The model under review builds one solid part; all positions refer to its coordinate system, in mm. Give positions to 0.01 mm unless a question says otherwise; leave off trailing zeros. Loops run counter-clockwise (first coordinate to the right, second up) from the corner with the lowest first, then second, coordinate; pieces in that order, holes last. Notation, with made-up numbers: M 66,74 L 100,74 A20 ccw 100,105 Z; hole C 30,13.5 d8. An arc over 180 degrees is marked long. One line per item, written item: value. Start each with the question number.
Q1. For pin 1 (1.5 mm diameter, centred on y = 34.5, z = 1.5, fed in from +X), flat-tipped, find the tip position at first contact; note if it passes through.
Q2. We need section A-A on x = 0. Write out the cut boundary in (y, z), plus the area to 3 significant figures.
Q3. We need section D-D on x = -13. Write out the cut boundary in (y, z).
Q4. To check wall thickness, follow line 1 along Y through (x, z) = (0, 2.95); line 2 along X through (y, z) = (-14, 0.55); line 3 along X through (y, z) = (-11.5, 1.2). State the ranges of each line that lie inside material, in increasing order. Write a range as from..to.
Q5. We need section B-B on x = 39. Write out the cut boundary in (y, z), plus the area to 3 significant figures.
Q6. We need section C-C on y = -24.5. Write out the cut boundary in (x, z), plus the area to 3 significant figures.
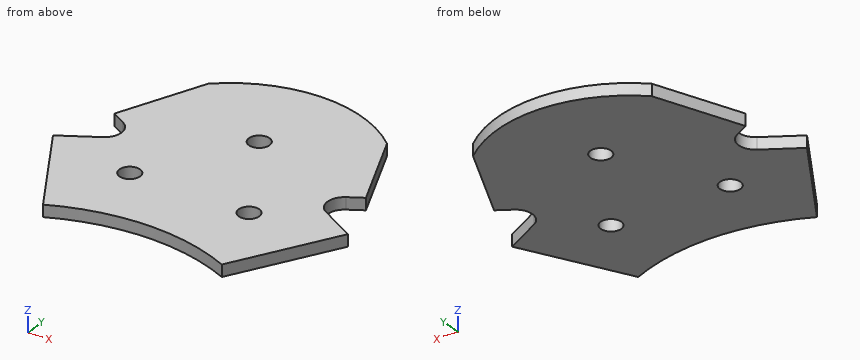
```python
from build123d import *

# Parameters (mm, degrees)
SKETCH1_R           = 3.5
BOSS_EXTRUDE1_DEPTH = 4


with BuildPart() as part:
    # Sketch1 → Boss-Extrude1 (new body)
    with BuildSketch(Plane.XY):
        with BuildLine():
            Line((-30, -39.805989232), (-49.472997898, -6.077767497))
            Line((-49.472997898, -6.077767497), (-37.435244785, 0.872232503))
            ThreePointArc((-37.435244785, 0.872232503), (-34.548493439, 5.872232503), (-37.435244785, 10.872232503))
            Line((-37.435244785, 10.872232503), (-42.198384506, 13.622232503))
            Line((-42.198384506, 13.622232503), (-30, 42.12134504))
            ThreePointArc((-30, 42.12134504), (0, 53.594010768), (30, 42.12134504))
            Line((30, 42.12134504), (42.198384506, 13.622232503))
            Line((42.198384506, 13.622232503), (37.435244785, 10.872232503))
            ThreePointArc((37.435244785, 10.872232503), (34.548493439, 5.872232503), (37.435244785, 0.872232503))
            Line((37.435244785, 0.872232503), (49.472997898, -6.077767497))
            Line((49.472997898, -6.077767497), (30, -39.805989232))
            ThreePointArc((30, -39.805989232), (0, -33.105989232), (-30, -39.805989232))
        make_face()
        with Locations((0, 23.094010768)):
            Circle(SKETCH1_R, mode=Mode.SUBTRACT)
        with Locations((-20, -11.547005384)):
            Circle(SKETCH1_R, mode=Mode.SUBTRACT)
        with Locations((20, -11.547005384)):
            Circle(SKETCH1_R, mode=Mode.SUBTRACT)
    extrude(amount=BOSS_EXTRUDE1_DEPTH)


solid = part.part
```
Solved:
1. pin 1: x = 33.58
2. outline: M -33.11,0 L 19.59,0 L 19.59,4 L -33.11,4 Z; M 26.59,0 L 53.59,0 L 53.59,4 L 26.59,4 Z
2. area: 319 mm2
3. outline: M -34.31,0 L 51.67,0 L 51.67,4 L -34.31,4 Z
4. line 1: -33.11..19.59, 26.59..53.59
4. line 2: -44.9..-22.5, -17.5..17.5, 22.5..44.9
4. line 3: -46.34..-23.5, -16.5..16.5, 23.5..46.34
5. outline: M -24.22,0 L -0.03,0 L -0.03,4 L -24.22,4 Z; M 11.78,0 L 21.09,0 L 21.09,4 L 11.78,4 Z
5. area: 134 mm2
6. outline: M -38.84,0 L 38.84,0 L 38.84,4 L -38.84,4 Z
6. area: 311 mm2
